```python
from build123d import *

# Parameters (mm, degrees)
SM_BASE_FLANGE_1_DEPTH           = 1.9
SM_EDGE_FLANGE_1_STRIP_W         = 9.0732
SM_EDGE_FLANGE_1_STRIP_H         = 1.9
SM_EDGE_FLANGE_1_STRIP_CUT_DEPTH = 60
SM_EDGE_FLANGE_1_DEPTH           = 60
CUT_EXTRUDE_1_DEPTH              = 88.336189521
SKETCH_9_R                       = 2.1
SKETCH_9_R_2                     = 1.6
SKETCH_9_R_3                     = 3.75
CUT_EXTRUDE_2_DEPTH              = 88.336189521
EXTRUDE_START                    = 1.9
SKETCH_10_R                      = 4.2
SKETCH_10_R_2                    = 2.1
EXTRUDE_2_DEPTH                  = 1.9
SKETCH_11_R                      = 1.6
SKETCH_11_R_2                    = 10
CUT_EXTRUDE_3_DEPTH              = 88.336189521


# Sheet-metal steps are written as plain solids
with BuildPart() as part:
    # Sketch 1 → 基体-法兰1 (new body)
    with BuildSketch(Plane.XY):
        with BuildLine():
            Line((-22, 80), (22, 80))
            ThreePointArc((22, 80), (27.656854249, 77.656854249), (30, 72))
            Line((30, 72), (30, 0))
            Line((30, 0), (-30, 0))
            Line((-30, 0), (-30, 72))
            ThreePointArc((-30, 72), (-27.656854249, 77.656854249), (-22, 80))
        make_face()
    extrude(amount=-SM_BASE_FLANGE_1_DEPTH)

    # 边线-法兰1 strip (across the edge) → 边线-法兰1 strip cut (cut)
    with BuildSketch(Plane.YZ.offset(-30)):
        with Locations((-3.8, -0.95)):
            Rectangle(SM_EDGE_FLANGE_1_STRIP_W, SM_EDGE_FLANGE_1_STRIP_H)
    extrude(amount=SM_EDGE_FLANGE_1_STRIP_CUT_DEPTH, mode=Mode.SUBTRACT)

    # 边线-法兰1 section (across the edge) → 边线-法兰1 (add)
    with BuildSketch(Plane.YZ.offset(-30)):
        with BuildLine():
            Line((-1.9, 0.7366), (-1.9, 18.1))
            Line((-1.9, 18.1), (0, 18.1))
            Line((0, 18.1), (0, 0.7366))
            ThreePointArc((0, 0.7366), (0.215745145, 0.215745145), (0.7366, 0))
            Line((0.7366, 0), (0.7366, -1.9))
            ThreePointArc((0.7366, -1.9), (-1.127757739, -1.127757739), (-1.9, 0.7366))
        make_face()
    extrude(amount=SM_EDGE_FLANGE_1_DEPTH)

    # 草图8 → 切除-拉伸1 (cut, through all)
    with BuildSketch(Plane(origin=(0, 0, 0), x_dir=(1, 0, 0), z_dir=(0, 1, 0))):
        Polygon((-30, -15.1), (-27, -18.1), (-30, -18.1), align=None)
        Polygon((27, -18.1), (30, -15.1), (30, -18.1), align=None)
    extrude(amount=-CUT_EXTRUDE_1_DEPTH, mode=Mode.SUBTRACT)

    # 草图9 → 切除-拉伸2 (cut, through all)
    with BuildSketch(Plane(origin=(0, 0, 0), x_dir=(1, 0, 0), z_dir=(0, 1, 0))):
        with Locations(Location((-25, -10, 0), (0, 0, 270))):
            Circle(SKETCH_9_R)
        with Locations(Location((-9, -10, 0), (0, 0, 270))):
            Circle(SKETCH_9_R_2)
        with Locations(Location((0, -10, 0), (0, 0, 270))):
            Circle(SKETCH_9_R_3)
        with Locations(Location((9, -10, 0), (0, 0, 270))):
            Circle(SKETCH_9_R_2)
        with Locations(Location((25, -10, 0), (0, 0, 270))):
            Circle(SKETCH_9_R)
    extrude(amount=-CUT_EXTRUDE_2_DEPTH, mode=Mode.SUBTRACT)

    # 草图10 → 凸台-拉伸2 (add)
    # profile 1 of 2: a face of its own
    with BuildSketch(Plane(origin=(0, 0, 0), x_dir=(1, 0, 0), z_dir=(0, 1, 0)).offset(EXTRUDE_START)):
        with Locations(Location((-25, -10, 0), (0, 0, 90))):
            Circle(SKETCH_10_R)
        with Locations(Location((-25, -10, 0), (0, 0, 270))):
            Circle(SKETCH_10_R_2, mode=Mode.SUBTRACT)
    # profile 2 of 2: a face of its own
    with BuildSketch(Plane(origin=(0, 0, 0), x_dir=(1, 0, 0), z_dir=(0, 1, 0)).offset(EXTRUDE_START)):
        with Locations(Location((25, -10, 0), (0, 0, 90))):
            Circle(SKETCH_10_R)
        with Locations(Location((25, -10, 0), (0, 0, 270))):
            Circle(SKETCH_10_R_2, mode=Mode.SUBTRACT)
    extrude(amount=-EXTRUDE_2_DEPTH)

    # 草图11 → 切除-拉伸3 (cut, through all)
    with BuildSketch(Plane.XY):
        with Locations((-17, 71.5)):
            Circle(SKETCH_11_R)
        with Locations((-17, 50)):
            Circle(SKETCH_11_R_2)
        with Locations((-17, 28.5)):
            Circle(SKETCH_11_R)
        with Locations((17, 28.5)):
            Circle(SKETCH_11_R)
        with Locations((17, 50)):
            Circle(SKETCH_11_R_2)
        with Locations((17, 71.5)):
            Circle(SKETCH_11_R)
    extrude(amount=-CUT_EXTRUDE_3_DEPTH, mode=Mode.SUBTRACT)


solid = part.part
```
Design review of the part built by this model. Coordinates are the model's own, in mm. A direction names the side the tool comes from. Give positions to 0.01 mm unless a question says otherwise; leave off trailing zeros. Order: outer loops, then holes, each group sorted by start corner. A loop starts at its lowest first (then second) coordinate and runs counter-clockwise, first axis right, second up. Notation, with made-up numbers: (33, 26.25) -> (76, 26.25) arc R15 ccw to (76, 41.25) -> close; hole circle Ø1 at (76.25, 9). An arc over 180 degrees is marked (long way). Write item = value, one per line. Start each with the question number.
(1) For pin 1 (2.5 mm diameter, centred on x = -17, y = 28.5, fed in from -Z); pin 2 (5 mm diameter, centred on x = 25, z = 10, fed in from +Y); pin 3 (4 mm diameter, centred on x = 17, y = 28.5, fed in from +Z), all flat-tipped, find the tip position at first contact; note any pin that passes through.
(2) For faces 1 (the face through (-23, 1.9, 8)), 2 (the face through (-30, 27, -0.3)), 3 (the face through (-28.54, 0.96, 7.74)), list the 3-axis set-ups (+Z, -Z, +X, -X, +Y, -Y) from which the entire face can be reached by the end or side of a thin tool; tool diameter is ignored.
(3) We need section C-C on x = 0. Write out the cut boundary in (y, z).
(4) Mouldability with a two-part tool opening along Z and no side actions: class faces 4 (the face through (-23.581, 0.027, 8.452)), 5 (the face through (28.5, -0.9, 16.6)), 6 (the face through (0, 80, -1)) as +Z half, -Z half, draft (parallel to the pull), parting line (faces both ways), or undercut.
(5) To check wall thickness, follow line 1 along X through (y, z) = (71.5, -1.05); line 2 along X through (y, z) = (-0.35, 10); line 3 along Y through (x, z) = (-17, -0.75). State the ranges of each line that lie inside material, in increasing order.
(6) We need section B-B on z = 10. State how many separate pieces and enclosed holes the cut face has, plus the area to 3 significant figures.
(7) We need section A-A on x = -17. Write out the cut boundary in (y, z).
(8) We need section D-D on y = 47.5. Write out the cut boundary in (x, z).
Numbers:
q1.pin_1 = through
q1.pin_2 = 1.9
q1.pin_3 = 0
q2.face_1 = +Z, +X, -X, +Y
q2.face_2 = +Z, -Z, -X, +Y, -Y
q2.face_3 = +Y
q3.outline = (-1.9, 0.74) arc R2.64 ccw to (0.74, -1.9) -> (80, -1.9) -> (80, 0) -> (0.74, 0) arc R0.74 cw to (0, 0.74) -> (0, 6.25) -> (-1.9, 6.25) -> close; (-1.9, 13.75) -> (0, 13.75) -> (0, 18.1) -> (-1.9, 18.1) -> close
q4.face_4 = undercut
q4.face_5 = +Z half
q4.face_6 = draft
q5.line_1 = -30 to -18.6, -15.4 to 15.4, 18.6 to 30
q5.line_2 = -30 to -27.1, -22.9 to -10.6, -7.4 to -3.75, 3.75 to 7.4, 10.6 to 22.9, 27.1 to 30
q5.line_3 = -1.44 to 26.9, 30.1 to 40, 60 to 69.9, 73.1 to 80
q6.separate_pieces = 6
q6.enclosed_holes = 0
q6.area = 87.6 mm^2
q7.outline = (-1.9, 0.74) arc R2.64 ccw to (0.74, -1.9) -> (26.9, -1.9) -> (26.9, 0) -> (0.74, 0) arc R0.74 cw to (0, 0.74) -> (0, 18.1) -> (-1.9, 18.1) -> close; (30.1, -1.9) -> (40, -1.9) -> (40, 0) -> (30.1, 0) -> close; (60, -1.9) -> (69.9, -1.9) -> (69.9, 0) -> (60, 0) -> close; (73.1, -1.9) -> (80, -1.9) -> (80, 0) -> (73.1, 0) -> close
q8.outline = (-30, -1.9) -> (-26.68, -1.9) -> (-26.68, 0) -> (-30, 0) -> close; (-7.32, -1.9) -> (7.32, -1.9) -> (7.32, 0) -> (-7.32, 0) -> close; (26.68, -1.9) -> (30, -1.9) -> (30, 0) -> (26.68, 0) -> close
